Autodesk Inventor part; units mm, degrees
ref_plane "YZ Plane" through (0, 0, 0) normal (1, 0, 0) x (0, 1, 0)
ref_plane "XZ Plane" through (0, 0, 0) normal (0, 1, 0) x (-1, 0, 0)
ref_plane "XY Plane" through (0, 0, 0) normal (0, 0, 1) x (1, 0, 0)
sketch "Sketch1" plane through (0, 0, 0) normal (0, 1, 0) x (-1, 0, 0)
  line L0 (0, 0) -> (-70, 0)
  line L1 (-70, 0) -> (-70, -50)
  line L2 (-70, -50) -> (0, -50)
  line L3 (0, -50) -> (0, 0)
  line L4 (0, -50) -> (0, -67.7966)
  line L5 (0, -67.7966) -> (-70, -50)
  dimension "d0" = 70
  dimension "d1" = 50
  dimension "d45" = 14.264
extrude "Extrusion1" add sketch "Sketch1" along normal blind 6
sketch "Sketch2" plane through (0, 6, 0) normal (0, 1, 0) x (1, 0, 0)
  line L0 (70, 50) -> (58.37, 52.9568) construction
  line L1 (70, 50) -> (0, 67.7966) construction
  line L2 (58.37, 52.9568) -> (52.555, 54.4352)
  line L3 (52.555, 54.4352) -> (53.2942, 57.3427)
  line L4 (53.2942, 57.3427) -> (59.1092, 55.8643)
  line L5 (59.1092, 55.8643) -> (58.37, 52.9568)
  line L6 (23.4799, 61.8271) -> (17.6649, 63.3055)
  line L7 (17.6649, 63.3055) -> (18.4041, 66.213)
  line L8 (18.4041, 66.213) -> (24.2191, 64.7346)
  line L9 (24.2191, 64.7346) -> (23.4799, 61.8271)
  point P0 (0, 0)
  dimension "d9" = 12
  dimension "d10" = 6
  dimension "d11" = 3
  dimension "d15" = 6
  dimension "d16" = 3
  dimension "d17" = 30
extrude "Extrusion2" add sketch "Sketch2" against normal blind 6
sketch "Sketch3" plane through (0, 6, 0) normal (0, 1, 0) x (1, 0, 0)
  line L0 (70, 0) -> (70, 50)
  line L1 (70, 54) -> (64, 54)
  line L2 (64, 54) -> (64, 41)
  line L3 (64, 41) -> (70, 41)
  line L4 (70, 41) -> (70, 54)
  line L5 (70, 0) -> (64, 0)
  line L6 (64, 0) -> (64, 9)
  line L7 (64, 9) -> (70, 9)
  line L8 (70, 9) -> (70, 0)
  line L9 (70, 35) -> (64, 35)
  line L10 (64, 35) -> (64, 15)
  line L11 (64, 15) -> (70, 15)
  line L12 (70, 15) -> (70, 35)
  point P0 (0, 0)
  dimension "d18" = 6
  dimension "d20" = 6
  dimension "d21" = 9
  dimension "d22" = 6
  dimension "d23" = 6
  dimension "d27" = 20
  dimension "d36" = 13
extrude "Extrusion3" cut sketch "Sketch3" along normal through all both and the other way through all
sketch "Sketch4" plane through (0, 6, 0) normal (0, 1, 0) x (1, 0, 0)
  line L0 (64, 0) -> (64, 9)
  line L1 (64, 6.25) -> (56, 6.25)
  line L2 (49, 6.25) -> (49, 3.75)
  line L3 (49, 3.75) -> (53.7, 3.75)
  line L4 (64, 3.75) -> (64, 6.25)
  line L5 (64, 9) -> (70, 9)
  line L6 (64, 43.75) -> (56, 43.75)
  line L7 (49, 43.75) -> (49, 46.25)
  line L8 (49, 46.25) -> (53.7, 46.25)
  line L9 (64, 46.25) -> (64, 43.75)
  line L10 (70, 41) -> (64, 41)
  line L11 (64, 41) -> (64, 51.5254)
  line L12 (56, 47.6) -> (53.7, 47.6)
  line L13 (53.7, 47.6) -> (53.7, 46.25)
  line L14 (53.7, 42.4) -> (56, 42.4)
  line L15 (56, 42.4) -> (56, 43.75)
  line L16 (53.7, 7.6) -> (56, 7.6)
  line L17 (56, 7.6) -> (56, 6.25)
  line L18 (56, 2.4) -> (53.7, 2.4)
  line L19 (53.7, 2.4) -> (53.7, 3.75)
  line L20 (53.7, 6.25) -> (53.7, 7.6)
  line L21 (53.7, 3.75) -> (53.7, 6.25) construction
  line L22 (56, 6.25) -> (56, 3.75) construction
  line L23 (56, 3.75) -> (56, 2.4)
  line L24 (56, 3.75) -> (64, 3.75)
  line L25 (53.7, 3.75) -> (56, 3.75) construction
  line L26 (56, 6.25) -> (53.7, 6.25) construction
  line L27 (53.7, 6.25) -> (49, 6.25)
  line L28 (53.7, 43.75) -> (53.7, 42.4)
  line L29 (53.7, 46.25) -> (53.7, 43.75) construction
  line L30 (53.7, 43.75) -> (49, 43.75)
  line L31 (56, 43.75) -> (53.7, 43.75) construction
  line L32 (56, 46.25) -> (56, 47.6)
  line L33 (56, 43.75) -> (56, 46.25) construction
  line L34 (53.7, 46.25) -> (56, 46.25) construction
  line L35 (56, 46.25) -> (64, 46.25)
  line L36 (6, 10) -> (12, 10)
  line L37 (12, 10) -> (12, 16)
  line L38 (12, 16) -> (6, 16)
  line L39 (6, 16) -> (6, 10)
  line L40 (6, 31) -> (12, 31)
  line L41 (12, 31) -> (12, 37)
  line L42 (12, 37) -> (6, 37)
  line L43 (6, 37) -> (6, 31)
  line L44 (0, 0) -> (64, 0)
  line L45 (0, 67.7966) -> (0, 0)
  point P0 (64, 45)
  dimension "d37" = 15
  dimension "d38" = 2.5
  dimension "d42" = 15
  dimension "d43" = 2.5
  dimension "d44" = 2.75
  dimension "d46" = 2.75
  dimension "d47" = 5.2
  dimension "d48" = 2.3
  dimension "d49" = 5.2
  dimension "d50" = 8
  dimension "d51" = 8
  dimension "d52" = 6
  dimension "d53" = 6
  dimension "d54" = 6
  dimension "d55" = 6
  dimension "d56" = 10
  dimension "d57" = 6
  dimension "d58" = 15
extrude "Extrusion4" cut sketch "Sketch4" along normal through all both and the other way through all
equation "\"d15\" = d10"
equation "\"d16\" = d11"
equation "\"d18\" = d20"
equation "\"d42\" = d37"
equation "\"d43\" = d38"
equation "\"d44\" = d46"
equation "\"d50\" = d51"
equation "\"d54\" = d52"
properties part number "pinball-case-left-wal-scaledl"
Read the model definition and answer for the solid it produces. Units are mm, in the model's axes. A direction names the side the tool comes from. Coordinates: 2 decimals unless noted, no trailing zeros. Loops run counter-clockwise (first coordinate to the right, second up) from the corner with the lowest first, then second, coordinate; pieces in that order, holes last.
Q1. Which of the six approach directions +Z, -Z, +X, -X, +Y, -Y give full straight-line access (tool end or side, diameter ignored) to faces 4 (the face through (64, 3, -49)), 5 (the face through (55, 3, -7.6)), 6 (the face through (28, 6, -33)), 7 (the face through (18.03, 3.04, -64.74)), 8 (the face through (51, 3, -46.25))?
Q2. The part is cut by section A-A on x = 60.5. Write down the section's boundary in (y, z), and give its area (3 significant figures).
Q3. Each of these flat-tipped pins is pushed along its axis until it touches: pin 1 Ø1.8 at (x, y) = (8.5, 3.5) entering from -Z; pin 2 Ø1.8 at (x, y) = (68.5, 1.5) entering from +Z; pin 3 Ø0.8 at (y, z) = (2, -45.5) entering from +X. Where does it stop, or does it pass through?
Q4. The part is cut by section B-B on z = -22.5. Write down the section's boundary in (x, y), and give its area (3 significant figures).
Q5. Consider probe 1 along X at (y, z) = (4.7, -35.5); probe 2 along Z at (x, y) = (66, 4.2); probe 3 along Z at (x, y) = (55.5, 1.55). Determine where each line is inside the solid, lowest interval first.
Q6. The part is cut by section C-C on y = 0.9. Give the number of separate pieces and of enclosed holes in the cut face, and give its area (3 significant figures).
Q7. The mould has two halves that part along X. Classify faces 1 (the face through (23.855, 3.042, -63.301)), 2 (the face through (51, 3, -3.75)), 3 (the face through (9, 3, -37)): +X half, -X half, draft (parallel to the pull), parting line (faces both ways), or undercut.
Q8. The part is cut by section D-D on x = 44. Write down the section's boundary in (y, z).
Results below:
1. face 4: -Z, +X, +Y, -Y
1. face 5: +Y, -Y
1. face 6: +Z, -Z, +X, -X, +Y
1. face 7: -Z, +Y, -Y
1. face 8: +X, +Y, -Y
2. outline: (0, -52.42) - (6, -52.42) - (6, -46.25) - (0, -46.25) - close; (0, -43.75) - (6, -43.75) - (6, -6.25) - (0, -6.25) - close; (0, -3.75) - (6, -3.75) - (6, 0) - (0, 0) - close
2. area: 284 mm2
3. pin 1: stops at z = -65.86
3. pin 2: stops at z = -9
3. pin 3: stops at x = 49
4. outline: (0, 0) - (64, 0) - (64, 6) - (0, 6) - close
4. area: 384 mm2
5. probe 1: x = 0 to 6, 12 to 70
5. probe 2: z = -41 to -35, -15 to -9
5. probe 3: z = -56.78 to -47.6, -42.4 to -7.6, -2.4 to 0
6. separate pieces: 1
6. enclosed holes: 2
6. area: 3,770 mm2
7. face 1: +X half
7. face 2: draft
7. face 3: undercut
8. outline: (0, -56.61) - (6, -56.61) - (6, 0) - (0, 0) - close
